Study the drawing (mm; zero at the part's minimum x, y, z) and answer. A direction names the side the tool comes from. Coordinates: 2 decimals unless noted, no trailing zeros. Order: outer loops, then holes, each group sorted by start corner. A loop starts at its lowest first (then second) coordinate and runs counter-clockwise, first axis right, second up.
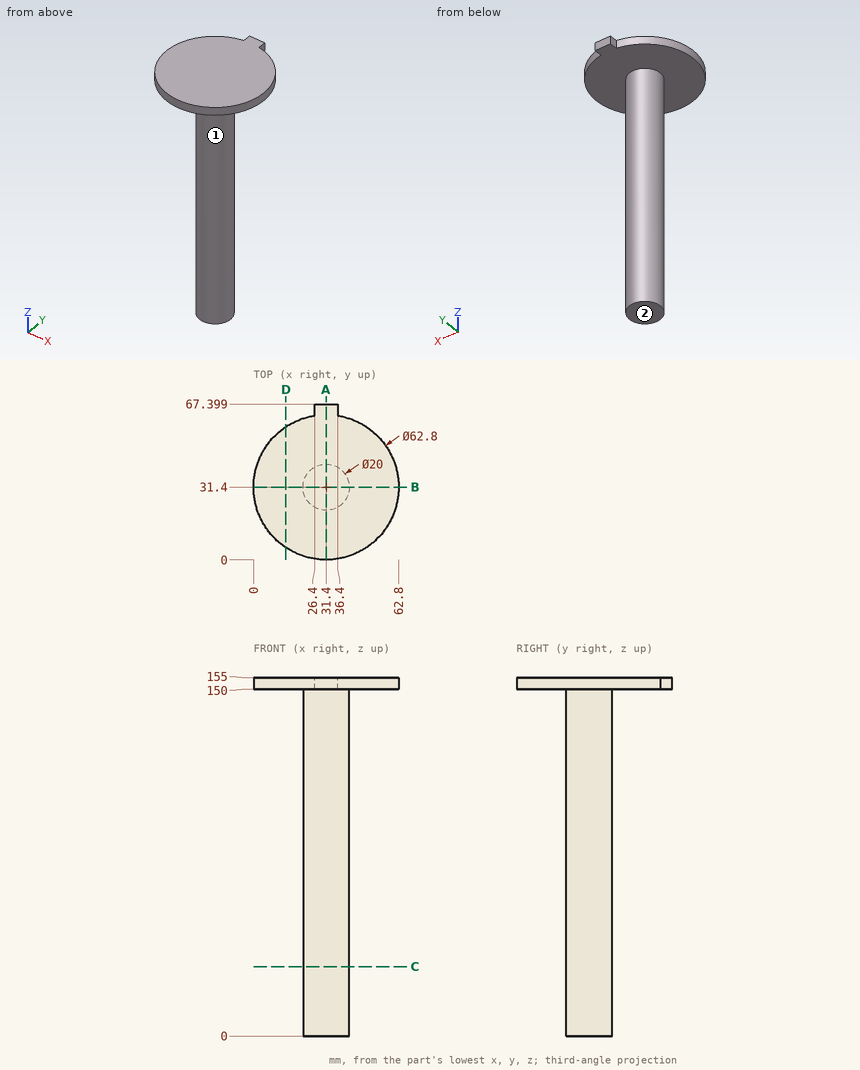
(1) For the marked faces 1 and 2, determine the directions among +Z, -Z, +X, -X, +Y, -Y from which every point of the face is accessible in a straight line to the end or side of a thin tool.
(2) Consider line 1 (Z direction, x = 28.5, y = 59); line 2 (X direction, y = 26.5, z = 94); line 3 (X direction, y = 25.5, z = 67) (1 decimal). Determine where each line is inside the solid, lowest interval first.
(3) Find section B-B (y = 31.4). Write down the section's boundary in (x, z).
(4) Find section A-A (x = 31.4). Write down the section's boundary in (y, z).
(5) Each of these flat-tipped pins is pushed along its axis until it touches: pin 1 Ø6 at (y, z) = (30, 129.5) entering from +X; pin 2 Ø2.5 at (y, z) = (64, 153.5) entering from +X; pin 3 Ø6 at (x, y) = (9, 20) entering from -Z; pin 4 Ø1.5 at (y, z) = (19, 130.5) entering from -X. Where does it stop, or does it pass through?
(6) Find section C-C (z = 30). Write down the section's boundary in (x, y), and give its area (3 significant figures).
(7) Find section D-D (x = 14). Write down the section's boundary in (y, z).
Findings below:
1. face 1: -Z
1. face 2: -Z, +X, -X, +Y, -Y
2. line 1: z = 150 to 155
2. line 2: x = 22.68 to 40.12
2. line 3: x = 23.3 to 39.5
3. outline: (0, 150) - (21.4, 150) - (21.4, 0) - (41.4, 0) - (41.4, 150) - (62.8, 150) - (62.8, 155) - (0, 155) - close
4. outline: (0, 150) - (21.4, 150) - (21.4, 0) - (41.4, 0) - (41.4, 150) - (67.4, 150) - (67.4, 155) - (0, 155) - close
5. pin 1: stops at x = 41.4
5. pin 2: stops at x = 36.4
5. pin 3: stops at z = 150
5. pin 4: passes through
6. outline: circle Ø20 at (31.4, 31.4)
6. area: 314 mm2
7. outline: (5.26, 150) - (57.54, 150) - (57.54, 155) - (5.26, 155) - close
